from build123d import *

# Parameters (mm, degrees)
EXTRUDE_1_DEPTH     = 2200
CUT_EXTRUDE_1_DEPTH = 46


with BuildPart() as part:
    # Эскиз1 → Вытянуть-Тонкостенный1 (new body)
    with BuildSketch(Plane(origin=(0, 0, 0), x_dir=(1, 0, 0), z_dir=(0, 1, 0))):
        Polygon((0, 45), (0, 0), (45, 0), (45, 5), (5, 5), (5, 45), align=None)
    extrude(amount=EXTRUDE_1_DEPTH)

    # Эскиз2 → Вырез-Вытянуть1 (cut, through all)
    with BuildSketch(Plane.ZY):
        Polygon((0, 0), (-45, 45), (-45, 0), align=None)
        Polygon((-45, 2200), (0, 2200), (-45, 2155), align=None)
    extrude(amount=-CUT_EXTRUDE_1_DEPTH, mode=Mode.SUBTRACT)


solid = part.part
Here's how the part is built. I have some questions about the finished solid (model axes, mm). A direction names the side the tool comes from. Round coordinates to 2 decimals unless told otherwise and drop trailing zeros. Order: outer loops, then holes, each group sorted by start corner. A loop starts at its lowest first (then second) coordinate and runs counter-clockwise, first axis right, second up. Notation, with made-up numbers: (-26, -37.5) -> (-7, -37.5) arc R12 ccw to (-7, -31.5) -> close; hole circle Ø7 at (80.5, 3.5). An arc over 180 degrees is marked (long way). Return JSON: item names as keys, results as strings.
Q1. If we mould it in two halves opening along Z, with no side actions, what happens to faces 1 (the flat face through (5, 1085, -25)), 2 (the flat face through (22, 1085, 0)), 3 (the flat face through (4, 12, -12))? For each: released by +Z, released by -Z, zero draft, split by the parting line, or undercut.
Filled sheet:
{"face 1": "zero draft", "face 2": "released by +Z", "face 3": "released by -Z"}
Q2. If we section it at B-B on y = 1490.5: List the corners of the cut face in (x, z) for me.
Filled sheet:
{"outline": "(0, -45) -> (5, -45) -> (5, -5) -> (45, -5) -> (45, 0) -> (0, 0) -> close"}
Q3. I need wall thicknesses on line 1 along X through (y, z) = (942, -19.5); line 2 along Z through (x, y) = (34.5, 776.5). Which ranges of each line are inside material? Lowest first, please. Write a range as from..to.
Filled sheet:
{"line 1": "x = 0..5", "line 2": "z = -5..0"}
Q4. If we section it at A-A on z = -16.5: List the corners of the cut face in (x, y) for me, plus the area to 3 significant figures.
Filled sheet:
{"outline": "(0, 16.5) -> (5, 16.5) -> (5, 2183.5) -> (0, 2183.5) -> close", "area": "10,800 mm^2"}
Q5. For pin 1 Ø20 at (y, z) = (1496, -22.5) entering from +X; pin 2 Ø5 at (x, z) = (27.5, -6.5) entering from -Y, each with a flat end and sliding along its axis, tell me the tip position at first contact or that it passes through.
Filled sheet:
{"pin 1": "stops at x = 5", "pin 2": "stops at y = 4"}
Q6. If we section it at C-C on x = 24: List the corners of the cut face in (y, z) for me, plus the area to 3 significant figures.
Filled sheet:
{"outline": "(0, 0) -> (5, -5) -> (2195, -5) -> (2200, 0) -> close", "area": "11,000 mm^2"}
Q7. Which directions (+Z, -Z, +X, -X, +Y, -Y) give clear straight access to the entire face, cutting with the end or side of a thin tool? Please do faces 4 (the flat face through (0, 1085, -23)), 5 (the flat face through (25, 1085, -5)).
Filled sheet:
{"face 4": "+Z, -Z, -X, +Y, -Y", "face 5": "-Z, +X, +Y, -Y"}
